Check sheet for the drawn part. Datum: minimum x, y, z corner. Units: mm. A direction names the side the tool comes from. Coordinates: 2 decimals unless noted, no trailing zeros. Loops run counter-clockwise (first coordinate to the right, second up) from the corner with the lowest first, then second, coordinate; pieces in that order, holes last.
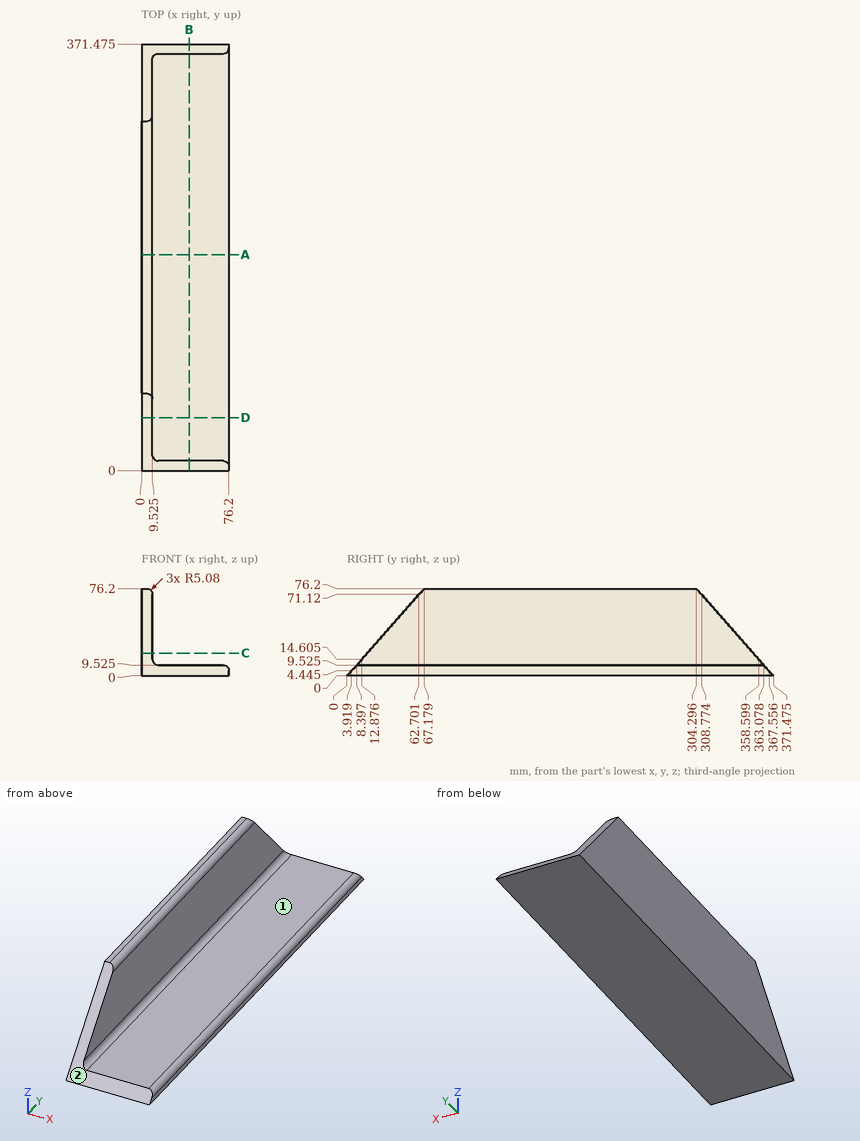
1) Section check C-C on z = 20. Enter the section's corners in (x, y) (1 decimal), plus the area to 3 significant figures.
Answer sheet:
outline: (0, 17.6) - (9.5, 17.6) - (9.5, 353.8) - (0, 353.8) - close
area: 3,200 mm2
2) Set-up check for the marked faces 1 and 2: record each of +Z, -Z, +X, -X, +Y, -Y from which the full face is reachable in a straight line by a thin tool's end or side.
Answer sheet:
face 1: +Z, +X, +Y, -Y
face 2: +Z, +X, -X, -Y
3) Depth check by flat-ended pin: pin 1 (5 mm diameter, centred on y = 148, z = 66.5, fed in from +X) (3 decimals); pin 2 (17 mm diameter, centred on x = 52.5, y = 177, fed in from +Z) (3 decimals); pin 3 (12 mm diameter, centred on x = 14.5, z = 20, fed in from +Y). Enter the tip coordinate at first touch or a pass-through.
Answer sheet:
pin 1: stops at x = 9.525
pin 2: stops at z = 9.525
pin 3: stops at y = 356.8
4) Scan lines: line 1 (X direction, y = 93.5, z = 32) (1 decimal); line 2 (Z direction, x = 14, y = 50). Record each from-to range of solid material in increasing order.
Answer sheet:
line 1: x = 0 to 9.5
line 2: z = 0 to 9.56
5) Section check B-B on x = 41.5. Enter the section's corners in (y, z) (1 decimal), plus the area to 3 significant figures.
Answer sheet:
outline: (0, 0) - (371.5, 0) - (363.1, 9.5) - (8.4, 9.5) - close
area: 3,460 mm2
6) Section check A-A on y = 188. Enter the section's corners in (x, z) (1 decimal).
Answer sheet:
outline: (0, 0) - (76.2, 0) - (76.2, 4.4) arc R5.1 ccw to (71.1, 9.5) - (14.6, 9.5) arc R5.1 cw to (9.5, 14.6) - (9.5, 71.1) arc R5.1 ccw to (4.4, 76.2) - (0, 76.2) - close
7) Section check D-D on y = 46. Enter the section's corners in (x, z) (1 decimal), plus the area to 3 significant figures.
Answer sheet:
outline: (0, 0) - (76.2, 0) - (76.2, 4.4) arc R5.1 ccw to (71.1, 9.5) - (14.6, 9.5) arc R5.1 cw to (9.5, 14.6) - (9.5, 52.2) - (0, 52.2) - close
area: 1,130 mm2
